Geometry check sheet. Reference: the model listing, model coordinates, mm. A direction names the side the tool comes from. Give positions to 0.01 mm unless a question says otherwise; leave off trailing zeros. Write each loop counter-clockwise with the first axis right and the second up, starting at its lowest first coordinate (ties: lowest second). Pieces come first, ordered by that corner, then holes. Notation, with made-up numbers: (73.5, -9) - (101.5, -9) arc R34 ccw to (101.5, 21) - close; hole circle Ø7 at (77, 42). An arc over 180 degrees is marked (long way). Write item = value, one per line. Start each with the question number.
(1) Thickness scan on L1, parallel to Z at x = -0.2, y = 0.25 (3 decimals); L2, parallel to Z at x = -0.6, y = 5 (3 decimals); L3, parallel to X at y = 5.75, z = 0. Record the ranges inside material, lowest first.
(2) Depth check by flat-ended pin: pin 1 Ø0.9 at (x, z) = (-0.5, 0.5) entering from +Y. Enter the tip coordinate at first touch or a pass-through.
(3) Section check D-D, the plane y = 4.5. Enter the section's corners in (x, z) (3 decimals).
(4) Section check B-B, the plane y = 0.75. Enter the section's corners in (x, z) (3 decimals).
(5) Access from +Z, -Z, +X, -X, +Y, -Y to the whole of each face (thin tool, end or side, straight path). Record for faces 1 (the flat face through (1, 4.4, 0.5)), 2 (the flat face through (0, 1, -0.5)), 3 (the flat face through (-1.27, 4, 0)).
(6) Section check A-A, the plane x = 0. Enter the section's corners in (y, z) (3 decimals), plus the area to 3 significant figures.
(7) Draft check along Y on faces 4 (the flat face through (0, 4, 1.27)), 5 (the flat face through (0, 4, -1)). Enter one of: pulls with the +Y half, pulls with the -Y half, needs draft (parallel to the pull), parting line crosses it, or undercut.
```python
from build123d import *

# Parameters (mm, degrees)
SKETCH1_W               = 2.54
SKETCH1_H               = 2.54
BOSS_EXTRUDE1_DEPTH     = 8.5
SHELL1_T                = -0.77
CHAMFER1_SIZE           = 0.5
CUT_EXTRUDE1_DEPTH      = 9.687680933
CUT_EXTRUDE1_DEPTH_BACK = 9.687680933
SKETCH2_W               = 1
SKETCH2_H               = 0.9
CUT_EXTRUDE3_START      = 1.4
SKETCH3_W               = 2
SKETCH3_H               = 2
CUT_EXTRUDE3_DEPTH      = 6
BOSS_EXTRUDE2_DEPTH     = 0.225


with BuildPart() as part:
    # Sketch1 → Boss-Extrude1 (new body)
    with BuildSketch(Plane(origin=(0, 0, 0), x_dir=(1, 0, 0), z_dir=(0, 1, 0))):
        Rectangle(SKETCH1_W, SKETCH1_H)
    extrude(amount=BOSS_EXTRUDE1_DEPTH)

    # Shell1
    shell1_openings = [part.faces().sort_by_distance(p)[0] for p in [
        (0, 8.5, 0),
    ]]
    offset(amount=SHELL1_T, openings=shell1_openings, kind=Kind.INTERSECTION)

    # Chamfer1
    chamfer1_edges = [part.edges().sort_by_distance(p)[0] for p in [
        (-0.5, 8.5, 0),
        (0, 8.5, 0.5),
        (0.5, 8.5, 0),
        (0, 8.5, -0.5),
    ]]
    chamfer(chamfer1_edges, length=CHAMFER1_SIZE)

    # Sketch2 → Cut-Extrude1 (cut, two sides: drawn at the far end of the back side and taken through both)
    with BuildSketch(Plane(origin=(0, 0, 0), x_dir=(0, 0, -1), z_dir=(1, 0, 0)).offset(-CUT_EXTRUDE1_DEPTH_BACK)):
        with Locations((0, 0.45)):
            Rectangle(SKETCH2_W, SKETCH2_H)
    extrude(amount=CUT_EXTRUDE1_DEPTH + CUT_EXTRUDE1_DEPTH_BACK, mode=Mode.SUBTRACT)

    # Sketch3 → Cut-Extrude3 (cut)
    with BuildSketch(Plane(origin=(0, 0, 0), x_dir=(1, 0, 0), z_dir=(0, 1, 0)).offset(CUT_EXTRUDE3_START)):
        Rectangle(SKETCH3_W, SKETCH3_H)
    extrude(amount=CUT_EXTRUDE3_DEPTH, mode=Mode.SUBTRACT)

    # Sketch4 → Boss-Extrude2 (add, symmetric)
    with BuildSketch(Plane.XY):
        with BuildLine():
            Line((-1, 7.3), (-1, 1.4))
            Line((-1, 1.4), (-0.325, 1.4))
            Line((-0.325, 1.4), (-0.325, -2.2))
            Line((-0.325, -2.2), (-0.215, -3))
            Line((-0.215, -3), (0.215, -3))
            Line((0.215, -3), (0.325, -2.2))
            Line((0.325, -2.2), (0.325, 1.4))
            Line((0.325, 1.4), (1, 1.4))
            Line((1, 1.4), (1, 7.3))
            ThreePointArc((1, 7.3), (0.931110636, 7.382586314), (0.837506501, 7.329628693))
            Line((0.837506501, 7.329628693), (0.6, 6.7))
            ThreePointArc((0.6, 6.7), (0.435896058, 5.8), (0.6, 4.9))
            Line((0.6, 4.9), (0.6, 2.8))
            ThreePointArc((0.6, 2.8), (0, 2.2), (-0.6, 2.8))
            Line((-0.6, 2.8), (-0.6, 4.9))
            ThreePointArc((-0.6, 4.9), (-0.435896058, 5.8), (-0.6, 6.7))
            Line((-0.6, 6.7), (-0.837506501, 7.329628693))
            ThreePointArc((-0.837506501, 7.329628693), (-0.931110636, 7.382586314), (-1, 7.3))
        make_face()
    extrude(amount=BOSS_EXTRUDE2_DEPTH, both=True)


solid = part.part
```
Model answer:
q1.L1 = -1.27 to -0.5, -0.225 to 0.225, 0.5 to 1.27
q1.L2 = -1.27 to -1, -0.225 to 0.225, 1 to 1.27
q1.L3 = -1.27 to -0.44, 0.44 to 1.27
q2.pin_1 = 8.45
q3.outline = (-1.27, -1.27) - (1.27, -1.27) - (1.27, 1.27) - (-1.27, 1.27) - close; hole (-1, -1) - (1, -1) - (1, -0.225) - (0.6, -0.225) - (0.6, 0.225) - (1, 0.225) - (1, 1) - (-1, 1) - (-1, 0.225) - (-0.6, 0.225) - (-0.6, -0.225) - (-1, -0.225) - close
q4.outline = (-1.27, -1.27) - (1.27, -1.27) - (1.27, -0.5) - (-1.27, -0.5) - close; (-1.27, 0.5) - (1.27, 0.5) - (1.27, 1.27) - (-1.27, 1.27) - close; (-0.325, -0.225) - (0.325, -0.225) - (0.325, 0.225) - (-0.325, 0.225) - close
q5.face_1 = none
q5.face_2 = -Y
q5.face_3 = +Z, -Z, -X, +Y, -Y
q6.outline = (-3, -0.225) - (2.2, -0.225) - (2.2, 0.225) - (-3, 0.225) - close; (0, -1.27) - (8.5, -1.27) - (8.5, -1) - (8, -0.5) - (7.4, -0.5) - (7.4, -1) - (1.4, -1) - (1.4, -0.5) - (0, -0.5) - close; (0, 0.5) - (1.4, 0.5) - (1.4, 1) - (7.4, 1) - (7.4, 0.5) - (8, 0.5) - (8.5, 1) - (8.5, 1.27) - (0, 1.27) - close
q6.area = 9.18 mm²
q7.face_4 = needs draft
q7.face_5 = undercut
